```python
from build123d import *

# Parameters (mm, degrees)
BOSS_EXTRUDE1_DEPTH = 0.95
SKETCH1_4_W         = 5
SKETCH1_4_H         = 4.2
BOSS_EXTRUDE2_DEPTH = 2.15
SKETCH3_W           = 6.9
SKETCH3_H           = 6.8
BOSS_EXTRUDE3_DEPTH = 4.83
SKETCH4_R           = 1.525
CUT_EXTRUDE1_DEPTH  = 3.15


with BuildPart() as part:
    # Sketch1 → Boss-Extrude1 (new body)
    with BuildSketch(Plane.XY):
        Polygon((-2.5, 15.5), (-7.125, 15.5), (-7.125, -15.5), (7.125, -15.5), (7.125, 15.5), (2.5, 15.5), align=None)
    extrude(amount=-BOSS_EXTRUDE1_DEPTH)

    # Sketch1<4> → Boss-Extrude2 (add, symmetric)
    with BuildSketch(Plane.XY):
        with Locations((0, 17.6)):
            Rectangle(SKETCH1_4_W, SKETCH1_4_H)
    extrude(amount=BOSS_EXTRUDE2_DEPTH, both=True)

    # Sketch3 → Boss-Extrude3 (add)
    with BuildSketch(Plane.XY):
        with Locations((3.675, 0.7)):
            Rectangle(SKETCH3_W, SKETCH3_H)
    extrude(amount=BOSS_EXTRUDE3_DEPTH)

    # Sketch4 → Cut-Extrude1 (cut, through all)
    with BuildSketch(Plane.XY):
        with Locations((0.3, -8.725)):
            Circle(SKETCH4_R)
    extrude(amount=-CUT_EXTRUDE1_DEPTH, mode=Mode.SUBTRACT)


solid = part.part
```
Input: part model. Units: mm. Frame: model coordinates. A direction names the side the tool comes from. Round coordinates to 2 decimals unless told otherwise and drop trailing zeros. Loops run counter-clockwise (first coordinate to the right, second up) from the corner with the lowest first, then second, coordinate; pieces in that order, holes last.
1) Set-up query: faces 1 (the flat face through (4.8, 15.5, -0.5)), 2 (the flat face through (0.225, 1, 2)), 3 (the flat face through (-2.5, 18, 0)), 4 (the flat face through (4, -2.7, 2)), 5 (the flat face through (0, 18, 2.15)). Return all of +Z, -Z, +X, -X, +Y, -Y with unobstructed straight access to the full face (end or side cutting, diameter ignored); none if empty.
Ans:
face 1: +Z, -Z, +X, +Y
face 2: +Z, -X, -Y
face 3: +Z, -Z, -X, +Y
face 4: +Z, +X, -X, -Y
face 5: +Z, +X, -X, +Y
2) Section query B-B on x = -2. Return the cut outline in (y, z), plus the area to 3 significant figures.
Ans:
outline: (-15.5, -0.95) - (15.5, -0.95) - (15.5, -2.15) - (19.7, -2.15) - (19.7, 2.15) - (15.5, 2.15) - (15.5, 0) - (-15.5, 0) - close
area: 47.5 mm2
3) Section query A-A on z = 1.5. Return the cut outline in (x, y) (3 decimals), plus the area to 3 significant figures.
Ans:
outline: (-2.5, 15.5) - (2.5, 15.5) - (2.5, 19.7) - (-2.5, 19.7) - close; (0.225, -2.7) - (7.125, -2.7) - (7.125, 4.1) - (0.225, 4.1) - close
area: 67.9 mm2
4) Section query C-C on y = 14.5. Return the cut outline in (x, z) (3 decimals).
Ans:
outline: (-7.125, -0.95) - (7.125, -0.95) - (7.125, 0) - (-7.125, 0) - close
5) Section query D-D on x = 4.75. Return the cut outline in (y, z), plus the area to 3 significant figures.
Ans:
outline: (-15.5, -0.95) - (15.5, -0.95) - (15.5, 0) - (4.1, 0) - (4.1, 4.83) - (-2.7, 4.83) - (-2.7, 0) - (-15.5, 0) - close
area: 62.3 mm2
6) Pin query (flat end, axial travel): pin 1 (1 mm diameter, centred on x = -0.5, y = 11, fed in from -Z); pin 2 (1.4 mm diameter, centred on y = 2, z = 2.5, fed in from -X) (3 decimals); pin 3 (0.6 mm diameter, centred on x = 0.5, z = 1.5, fed in from -Y). Return the tip coordinate at first contact, or that it passes through.
Ans:
pin 1: stops at z = -0.95
pin 2: stops at x = 0.225
pin 3: stops at y = -2.7
7) Material intervals for line 1 (Y direction, x = 2, z = 1.5); line 2 (Z direction, x = 2, y = 6); line 3 (Z direction, x = 2, y = 0.5), sorted ascending.
Ans:
line 1: y = -2.7 to 4.1, 15.5 to 19.7
line 2: z = -0.95 to 0
line 3: z = -0.95 to 4.83
8) Pull-direction query (X, two-part tool) for faces 6 (the cylindrical face through (1, -10.08, -0.47)), 7 (the flat face through (0, 0, -0.95)), 8 (the flat face through (-7.125, 0.2, -0.5)), 9 (the flat face through (2.5, 18, 0)); classes: released by +X, released by -X, zero draft, split by the parting line, or undercut.
Ans:
face 6: undercut
face 7: zero draft
face 8: released by -X
face 9: released by +X
